Read the model definition and answer for the solid it produces. Units are mm, in the model's axes. Face numbers are marked on the shaded views. A direction names the side the tool comes from. Coordinates: 2 decimals unless noted, no trailing zeros. Loops run counter-clockwise (first coordinate to the right, second up) from the corner with the lowest first, then second, coordinate; pieces in that order, holes last.
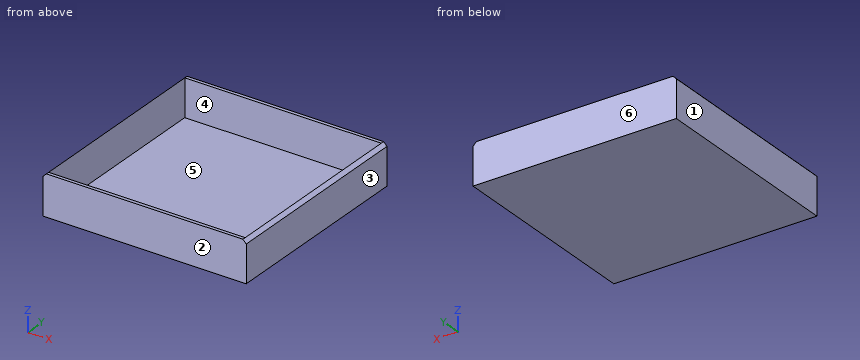
from build123d import *

# Parameters (mm, degrees)
F0_W     = 76.2
F0_H     = 76.2
F0_W_2   = 73.66
F0_H_2   = 73.66
F1_DEPTH = 13.97
F2_SIZE  = 1.26999
F3_W     = 76.2
F3_H     = 76.2
F4_DEPTH = 1.27


# Not quite as in the source:
# - a fillet or chamfer is up to 0.001 mm smaller than in the source, because OpenCascade refuses the exact size


with BuildPart() as f1:
    # F0 (on Top) → F1 (new body)
    with BuildSketch(Plane.XY):
        Rectangle(F0_W, F0_H)
        Rectangle(F0_W_2, F0_H_2, mode=Mode.SUBTRACT)
    extrude(amount=F1_DEPTH)

    # F2 (size 1.27 in the source; OpenCascade refuses exactly that, so slightly less here)
    f2_edges = [f1.edges().sort_by_distance(p)[0] for p in [
        (-38.1, 0, 13.97),
        (38.1, 0, 13.97),
    ]]
    chamfer(f2_edges, length=F2_SIZE)

    # F3 (on face) → F4 (join)
    with BuildSketch(Plane(origin=(0, 0, 0), x_dir=(1, 0, 0), z_dir=(0, 0, -1))):
        Rectangle(F3_W, F3_H)
    extrude(amount=F4_DEPTH)


solid = f1.part
Item 1: Find the intervals of material crossed by line 1 along Y through (x, z) = (-0.5, 10.25); line 2 along Z through (x, y) = (33, -14), in increasing order.
Numbers:
line 1: y = -38.1 to -36.83, 36.83 to 38.1
line 2: z = -1.27 to 0
Item 2: A cutting plane is placed at B-B on x = 21. Determine the outline of the cut face in (y, z).
Numbers:
outline: (-38.1, -1.27) - (38.1, -1.27) - (38.1, 13.97) - (36.83, 13.97) - (36.83, 0) - (-36.83, 0) - (-36.83, 13.97) - (-38.1, 13.97) - close
Item 3: Which of the six approach directions +Z, -Z, +X, -X, +Y, -Y give full straight-line access (tool end or side, diameter ignored) to the marked faces 5 and 6?
Numbers:
face 5: +Z
face 6: +Z, -Z, +X, -X, +Y
Item 4: Determine the mould class of the marked faces 1, 2, 3 and 4 for opening direction X: released by +X, released by -X, zero draft, split by the parting line, or undercut.
Numbers:
face 1: released by -X
face 2: zero draft
face 3: released by +X
face 4: undercut
Item 5: Given pin 1 (12 mm diameter, centred on x = -15.5, y = 9, fed in from +Z), flat-ended and moving along its own axis, determine where the tip first touches the part or whether it passes through.
Numbers:
pin 1: stops at z = 0
Item 6: A cutting plane is placed at A-A on z = 3.5. Determine the outline of the cut face in (x, y), then the cut area to 3 significant figures.
Numbers:
outline: (-38.1, -38.1) - (38.1, -38.1) - (38.1, 38.1) - (-38.1, 38.1) - close; hole (-36.83, -36.83) - (36.83, -36.83) - (36.83, 36.83) - (-36.83, 36.83) - close
area: 381 mm2
